```python
from build123d import *

# Parameters (mm, degrees)
F0_W     = 30
F0_H     = 40
F1_DEPTH = 20
F2_T     = -2.5
F3_W     = 25
F3_H     = 35
F4_DEPTH = 25
F4_TAPER = 25


with BuildPart() as f1:
    # F0 (on Top) → F1 (new body)
    with BuildSketch(Plane.XY):
        Rectangle(F0_W, F0_H)
    extrude(amount=F1_DEPTH)

    # F2
    f2_openings = [f1.faces().sort_by_distance(p)[0] for p in [
        (0, 0, 20),
    ]]
    offset(amount=F2_T, openings=f2_openings)

    # F3 (on face) → F4 (join)
    with BuildSketch(Plane.XY.offset(2.5)):
        Rectangle(F3_W, F3_H)
    extrude(amount=F4_DEPTH, taper=F4_TAPER)


solid = f1.part
```
Can you work these out from the model? Positions are in its coordinate system, mm. A direction names the side the tool comes from. Give positions to 0.01 mm unless a question says otherwise; leave off trailing zeros. Write each loop counter-clockwise with the first axis right and the second up, starting at its lowest first coordinate (ties: lowest second). Pieces come first, ordered by that corner, then holes. Notation, with made-up numbers: (52, 76.5) -> (79, 76.5) arc R20 ccw to (79, 109.5) -> close; hole circle Ø4 at (10, 30). An arc over 180 degrees is marked (long way). One line per item, written item: value.
Q1. Imagine slicing it at D-D on z = 13. Please give me the cut outline in (x, y), and give its area (3 significant figures).
Results found:
outline: (-15, -20) -> (15, -20) -> (15, 20) -> (-15, 20) -> close; (-7.6, -12.6) -> (7.6, -12.6) -> (7.6, 12.6) -> (-7.6, 12.6) -> close; hole (-12.5, -17.5) -> (12.5, -17.5) -> (12.5, 17.5) -> (-12.5, 17.5) -> close
area: 708 mm^2
Q2. Imagine slicing it at C-C on x = -9.75. Please give me the cut outline in (y, z), and give its area (3 significant figures).
Results found:
outline: (-20, 0) -> (20, 0) -> (20, 20) -> (17.5, 20) -> (17.5, 2.5) -> (14.75, 8.4) -> (-14.75, 8.4) -> (-17.5, 2.5) -> (-17.5, 20) -> (-20, 20) -> close
area: 378 mm^2
Q3. Imagine slicing it at A-A on z = 3.5. Please give me the cut outline in (x, y), and give its area (3 significant figures).
Results found:
outline: (-15, -20) -> (15, -20) -> (15, 20) -> (-15, 20) -> close; (-12.03, -17.03) -> (12.03, -17.03) -> (12.03, 17.03) -> (-12.03, 17.03) -> close; hole (-12.5, -17.5) -> (12.5, -17.5) -> (12.5, 17.5) -> (-12.5, 17.5) -> close
area: 1,140 mm^2
Q4. For P1, Ø12, axis at y = 2, z = 22.5, coming from the +X side; P2, Ø6, axis at x = -10.5, y = -8, coming from the +Z side, each with a flat end and sliding along its axis, tell me the tip position at first contact or that it passes through.
Results found:
P1: stops at x = 15
P2: stops at z = 20
Q5. Please list where these lines run through material, in increasing order: line 1 (Y direction, x = 5.5, z = 8.5); line 2 (X direction, y = 14.5, z = 8.25); line 3 (X direction, y = 15, z = 9). Write a range as [from, to].
Results found:
line 1: y = [-20, -17.5], [-14.7, 14.7], [17.5, 20]
line 2: x = [-15, -12.5], [-9.82, 9.82], [12.5, 15]
line 3: x = [-15, -12.5], [12.5, 15]
Q6. We'd pull the mould along Y, two halves only. Please class faces 1 (the face through (0, 20, 10)), 2 (the face through (15, 0, 10)), 3 (the face through (-8.048, -0.245, 12.047)), 4 (the face through (-0.175, 13.048, 12.047)): +Y half, -Y half, draft (parallel to the pull), parting line (faces both ways), or undercut.
Results found:
face 1: +Y half
face 2: draft
face 3: undercut
face 4: undercut
Q7. Imagine slicing it at B-B on y = 3. Please give me the cut outline in (x, z), and give its area (3 significant figures).
Results found:
outline: (-15, 0) -> (15, 0) -> (15, 20) -> (12.5, 20) -> (12.5, 2.5) -> (0.84, 27.5) -> (-0.84, 27.5) -> (-12.5, 2.5) -> (-12.5, 20) -> (-15, 20) -> close
area: 496 mm^2
Q8. Which directions (+Z, -Z, +X, -X, +Y, -Y) give clear straight access to the entire face, cutting with the end or side of a thin tool? Please do faces 5 (the face through (8.048, 0.245, 12.047)), 6 (the face through (-15, 0, 10)).
Results found:
face 5: +Z
face 6: +Z, -Z, -X, +Y, -Y
